Read the model definition and answer for the solid it produces. Units are mm, in the model's axes. A direction names the side the tool comes from. Give positions to 0.01 mm unless a question says otherwise; leave off trailing zeros. Loops run counter-clockwise (first coordinate to the right, second up) from the corner with the lowest first, then second, coordinate; pieces in that order, holes last. Notation, with made-up numbers: (-36.75, -38.75) - (-8.75, -38.75) arc R30 cw to (-8.75, -14.75) - close; hole circle Ø3 at (89, -35). An arc over 180 degrees is marked (long way). Put each result on its own line as item: value. Start each with the question number.
1. For faces 5 (the flat face through (-103, 60.3, 8)), 6 (the flat face through (-158, -4.7, -6)), 7 (the flat face through (-158, 65, -6)), 8 (the cylindrical face through (-139.866, -12.61, 17.484)), determine the directions among +Z, -Z, +X, -X, +Y, -Y from which every point of the face is accessible in a straight line to the end or side of a thin tool.
2. A cutting plane is placed at A-A, the plane y = 44.5. Determine the outline of the cut face in (x, z), plus the area to 3 significant figures.
3. A cutting plane is placed at D-D, the plane z = -4.3. Determine the outline of the cut face in (x, y).
4. A cutting plane is placed at B-B, the plane x = -111. Count the separate pieces of the cut face and the enclosed holes in it, plus the area to 3 significant figures.
5. For a pull along X with two mould halves and no side action, classify faces 1 (the flat face through (-111, 60, 0.8)), 2 (the flat face through (-100.01, 65.4, 10.88)), 3 (the flat face through (-150.9, 31, -4)), 4 (the flat face through (-159, 59, -3)) as released by +X, released by -X, zero draft, split by the parting line, or undercut.
6. A cutting plane is placed at C-C, the plane y = 5.2. Determine the outline of the cut face in (x, z), plus the area to 3 significant figures.
7. Consider L1, parallel to Y at x = -144.7, z = 0.95; L2, parallel to Y at x = -134, z = 20.5; L3, parallel to Y at x = -144, z = 1. Determine where each line is inside the solid, lowest interval first. Write a range as from..to.
8. Given pin 1 Ø1 at (y, z) = (60.5, 18) entering from -X; pin 2 Ø1.2 at (x, y) = (-102, 63) entering from +Z; pin 3 Ø7 at (x, z) = (-127.5, 9) entering from -Y; pin 4 Ø1.5 at (y, z) = (67, 11) entering from +X, each flat-ended and moving along its own axis, determine where each tip first touches the part or whether it passes through.
```python
from build123d import *

# Parameters (mm, degrees)
SKETCH_1_W          = 33.55
SKETCH_1_H          = 60.3
SKETCH_1_R          = 1.2
EXTRUDE_1_DEPTH     = 2
SKETCH_2_W          = 2
SKETCH_2_H          = 60.3
EXTRUDE_2_DEPTH     = 9.9
SKETCH_3_W          = 9.9
SKETCH_3_H          = 2
EXTRUDE_3_DEPTH     = 1.9
SKETCH_4_W          = 10.719852834
SKETCH_4_H          = 56.3
SKETCH_4_W_2        = 2
SKETCH_4_H_2        = 60.3
EXTRUDE_5_DEPTH     = 3
SKETCH_6_W          = 14.719852834
SKETCH_6_H          = 4.7
EXTRUDE_6_DEPTH     = 3
SKETCH_7_W          = 9.4
SKETCH_7_H          = 6
SKETCH_7_R          = 1.5
EXTRUDE_7_DEPTH     = 14.4
EXTRUDE_8_DEPTH     = 17.1
EXTRUDE_9_DEPTH     = 8.35
SKETCH_10_W         = 43.45
SKETCH_10_H         = 4
EXTRUDE_10_DEPTH    = 8.35
CUT_EXTRUDE_START   = -0.6
CUT_EXTRUDE_1_DEPTH = 0.6
CUT_EXTRUDE_2_DEPTH = 0.6
SKETCH_13_W         = 43.45
SKETCH_13_H         = 4
EXTRUDE_11_DEPTH    = 2
SKETCH_14_W         = 43.45
SKETCH_14_H         = 4
EXTRUDE_12_DEPTH    = 2
EXTRUDE_13_DEPTH    = 4
SKETCH_16_W         = 2.5
SKETCH_16_H         = 40
EXTRUDE_14_DEPTH    = 10
SKETCH_17_W         = 4
SKETCH_17_H         = 5.65
EXTRUDE_15_DEPTH    = 17.4
EXTRUDE_16_DEPTH    = 4
SKETCH_19_W         = 1.8
SKETCH_19_H         = 1.8
EXTRUDE_17_DEPTH    = 21.4
SKETCH_20_W         = 12.1
SKETCH_20_H         = 1.8
EXTRUDE_18_DEPTH    = 16
EXTRUDE_START       = -4
EXTRUDE_22_DEPTH    = 25.4
EXTRUDE_23_DEPTH    = 25.4
CUT_EXTRUDE_3_DEPTH = 21.4
EXTRUDE_24_DEPTH    = 4
EXTRUDE_25_DEPTH    = 21.4
SKETCH_26_W         = 1.445945033
SKETCH_26_H         = 2.5
EXTRUDE_26_DEPTH    = 10
EXTRUDE_27_DEPTH    = 21.4
EXTRUDE_28_DEPTH    = 21.4
SKETCH_29_W         = 21.4
SKETCH_29_H         = 5
EXTRUDE_29_DEPTH    = 3
SKETCH_30_R         = 1.2
CUT_EXTRUDE_4_DEPTH = 12
SKETCH_31_W         = 13.445945033
SKETCH_31_H         = 37.5
SKETCH_31_W_2       = 7.004054967
SKETCH_31_H_2       = 40
CUT_EXTRUDE_5_DEPTH = 2
CUT_EXTRUDE_START_2 = -9.4
CUT_EXTRUDE_6_DEPTH = 9.4
CHAMFER_2_SIZE      = 2
CHAMFER_3_SIZE      = 3
CHAMFER_4_SIZE      = 3


with BuildPart() as part:
    # 草图1 → 凸台-拉伸1 (new body)
    with BuildSketch(Plane.XY):
        with Locations((-131.125, 30.15)):
            Rectangle(SKETCH_1_W, SKETCH_1_H)
        with Locations((-144.7, 5.2)):
            Circle(SKETCH_1_R, mode=Mode.SUBTRACT)
        with Locations((-117.55, 5.2)):
            Circle(SKETCH_1_R, mode=Mode.SUBTRACT)
        with Locations((-117.55, 55.1)):
            Circle(SKETCH_1_R, mode=Mode.SUBTRACT)
        with Locations((-144.7, 55.1)):
            Circle(SKETCH_1_R, mode=Mode.SUBTRACT)
    extrude(amount=EXTRUDE_1_DEPTH)

    # 草图2 → 凸台-拉伸2 (add)
    with BuildSketch(Plane(origin=(-114.35, 0, 0), x_dir=(0, 0, -1), z_dir=(1, 0, 0))):
        with Locations((-1, 30.15)):
            Rectangle(SKETCH_2_W, SKETCH_2_H)
    extrude(amount=EXTRUDE_2_DEPTH)

    # 草图3 → 凸台-拉伸3 (add)
    with BuildSketch(Plane(origin=(0, 0, 0), x_dir=(-1, 0, 0), z_dir=(0, 0, -1))):
        with Locations((109.4, 59.3)):
            Rectangle(SKETCH_3_W, SKETCH_3_H)
        with Locations((109.4, 1)):
            Rectangle(SKETCH_3_W, SKETCH_3_H)
    extrude(amount=EXTRUDE_3_DEPTH)

    # 草图4 → 凸台-拉伸5 (add)
    with BuildSketch(Plane.ZY.offset(147.9)):
        Polygon((0, 60.3), (-12.719852834, 60.3), (-12.719852834, 58.3), (-2, 58.3), (-2, 2), (-12.719852834, 2), (-12.719852834, 0), (0, 0), align=None)
        with Locations((-7.359926417, 30.15)):
            Rectangle(SKETCH_4_W, SKETCH_4_H)
        with Locations((1, 30.15)):
            Rectangle(SKETCH_4_W_2, SKETCH_4_H_2)
    extrude(amount=EXTRUDE_5_DEPTH)

    # 草图6 → 凸台-拉伸6 (add)
    with BuildSketch(Plane.ZY.offset(150.9)):
        with Locations((-5.359926417, 62.65)):
            Rectangle(SKETCH_6_W, SKETCH_6_H)
        with Locations((-5.359926417, -2.35)):
            Rectangle(SKETCH_6_W, SKETCH_6_H)
    extrude(amount=-EXTRUDE_6_DEPTH)

    # 草图7 → 凸台-拉伸7 (add)
    # profile 1 of 2: a face of its own
    with BuildSketch(Plane.ZY.offset(150.9)):
        with Locations((-2.7, 62)):
            Rectangle(SKETCH_7_W, SKETCH_7_H)
        with Locations(Location((-4.3, 61.9, 0), (0, 0, 180))):
            Circle(SKETCH_7_R, mode=Mode.SUBTRACT)
    # profile 2 of 2: a face of its own
    with BuildSketch(Plane.ZY.offset(150.9)):
        with Locations((-2.7, -1.7)):
            Rectangle(SKETCH_7_W, SKETCH_7_H)
        with Locations(Location((-4.3, -1.6, 0), (0, 0, 180))):
            Circle(SKETCH_7_R, mode=Mode.SUBTRACT)
    extrude(amount=EXTRUDE_7_DEPTH)

    # 草图8 → 凸台-拉伸8 (add)
    with BuildSketch(Plane.ZY.offset(150.9)):
        Polygon((-7.8, 59), (-7.8, 1.3), (-7.4, 1.3), (-7.4, -4.7), (-12.719852834, -4.7), (-12.719852834, 65), (-7.4, 65), (-7.4, 59), align=None)
    extrude(amount=EXTRUDE_8_DEPTH)

    # 草图9 → 凸台-拉伸9 (add)
    with BuildSketch(Plane(origin=(0, 60.3, 0), x_dir=(1, 0, 0), z_dir=(0, 1, 0))):
        Polygon((-114.35, 1.9), (-114.35, 0), (-147.9, 0), (-147.9, -2), (-104.45, -2), (-104.45, 1.9), align=None)
        Polygon((-114.35, 1.9), (-104.45, 1.9), (-104.45, 2), (-147.9, 2), (-147.9, 0), (-114.35, 0), align=None)
    extrude(amount=EXTRUDE_9_DEPTH)

    # 草图10 → 凸台-拉伸10 (add)
    with BuildSketch(Plane.XZ):
        with Locations((-126.175, 0)):
            Rectangle(SKETCH_10_W, SKETCH_10_H)
    extrude(amount=EXTRUDE_10_DEPTH)

    # 草图11 → 切除-拉伸1 (cut)
    with BuildSketch(Plane.XY.offset(2).offset(CUT_EXTRUDE_START)):
        with BuildLine():
            Line((-104.45, 51.65), (-104.45, 67.75))
            Line((-104.45, 67.75), (-116.55, 67.75))
            Line((-116.55, 67.75), (-116.55, 55.763324958))
            ThreePointArc((-116.55, 55.763324958), (-116.354567134, 55.204595711), (-116.45, 54.620416848))
            Line((-116.45, 54.620416848), (-116.45, 51.65))
            Line((-116.45, 51.65), (-104.45, 51.65))
        make_face()
    extrude(amount=CUT_EXTRUDE_1_DEPTH, mode=Mode.SUBTRACT)

    # 草图12 → 切除-拉伸2 (cut)
    with BuildSketch(Plane.XY.offset(1.4)):
        with BuildLine():
            Line((-113.374176728, 54.65), (-107.45, 54.65))
            Line((-107.45, 54.65), (-107.45, 64.75))
            Line((-107.45, 64.75), (-113.55, 64.75))
            Line((-113.55, 64.75), (-113.55, 56.380624847))
            ThreePointArc((-113.55, 56.380624847), (-113.371508988, 55.524514858), (-113.374176728, 54.65))
        make_face()
    extrude(amount=-CUT_EXTRUDE_2_DEPTH, mode=Mode.SUBTRACT)

    # 草图13 → 凸台-拉伸11 (add)
    with BuildSketch(Plane(origin=(0, 68.65, 0), x_dir=(1, 0, 0), z_dir=(0, 1, 0))):
        with Locations((-126.175, 0)):
            Rectangle(SKETCH_13_W, SKETCH_13_H)
    extrude(amount=EXTRUDE_11_DEPTH)

    # 草图14 → 凸台-拉伸12 (add)
    with BuildSketch(Plane.XZ.offset(8.35)):
        with Locations((-126.175, 0)):
            Rectangle(SKETCH_14_W, SKETCH_14_H)
    extrude(amount=EXTRUDE_12_DEPTH)

    # 草图15 → 凸台-拉伸13 (add)
    with BuildSketch(Plane.XY.offset(2)):
        Polygon((-147.9, 70.65), (-165.3, 65), (-147.9, 65), align=None)
    extrude(amount=-EXTRUDE_13_DEPTH)

    # 草图16 → 凸台-拉伸14 (add)
    with BuildSketch(Plane.XY.offset(2)):
        with Locations((-142.645945033, 30.15)):
            Rectangle(SKETCH_16_W, SKETCH_16_H)
        with Locations((-119.145945033, 30.15)):
            Rectangle(SKETCH_16_W, SKETCH_16_H)
    extrude(amount=EXTRUDE_14_DEPTH)

    # 草图17 → 凸台-拉伸15 (add)
    with BuildSketch(Plane.ZY.offset(147.9)):
        with Locations((0, -7.525)):
            Rectangle(SKETCH_17_W, SKETCH_17_H)
    extrude(amount=EXTRUDE_15_DEPTH)

    # 草图18 → 凸台-拉伸16 (add)
    with BuildSketch(Plane.XY.offset(2)):
        Polygon((-104.45, 67.75), (-104.45, 60.3), (-95.7, 60.3), (-104.45, 70.65), align=None)
        Polygon((-104.45, 0), (-104.45, -10.35), (-95.7, 0), align=None)
    extrude(amount=-EXTRUDE_16_DEPTH)

    # 草图19 → 凸台-拉伸17 (add)
    with BuildSketch(Plane.XY.offset(2)):
        Polygon((-165.3, 65), (-159.471717964, 65), (-147.615080796, 68.85), (-118.35, 68.85), (-118.35, 70.65), (-147.9, 70.65), align=None)
        with Locations((-117.45, 69.75)):
            Rectangle(SKETCH_19_W, SKETCH_19_H)
        Polygon((-95.7, 60.3), (-104.45, 70.65), (-104.45, 67.861945247), (-102.65, 65.73280239), (-99.57879025, 62.1), (-99.57879025, 60.3), align=None)
        Polygon((-105.285311989, -8.55), (-163.5, -8.55), (-165.3, -8.55), (-165.3, -10.35), (-104.45, -10.35), (-95.7, 0), (-99.57879025, 0), (-99.57879025, -1.8), align=None)
    extrude(amount=EXTRUDE_17_DEPTH)

    # 草图20 → 凸台-拉伸18 (add)
    with BuildSketch(Plane.XY.offset(23.4)):
        with Locations((-110.5, 69.75)):
            Rectangle(SKETCH_20_W, SKETCH_20_H)
    extrude(amount=-EXTRUDE_18_DEPTH)

    # 草图21 → 凸台-拉伸22 (add)
    with BuildSketch(Plane.XY.offset(2).offset(EXTRUDE_START)):
        Polygon((-165.3, -8.55), (-165.3, -4.7), (-168, -4.7), (-165.3, -10.35), align=None)
    extrude(amount=EXTRUDE_22_DEPTH)

    # 草图22 → 凸台-拉伸23 (add)
    with BuildSketch(Plane.XY.offset(23.4)):
        Polygon((-163.305030212, -10.35), (-165.3, -10.35), (-162.432743363, -16.35), (-141.174369577, -16.35), (-137.174369577, -10.35), (-138.374369577, -10.35), (-141.174369577, -14.55), (-161.297950566, -14.55), align=None)
    extrude(amount=-EXTRUDE_23_DEPTH)

    # 草图23 → 切除-拉伸3 (cut)
    with BuildSketch(Plane.XY.offset(23.4)):
        Polygon((-164.165207203, -8.55), (-163.305030212, -10.35), (-138.374369577, -10.35), (-137.174369577, -8.55), align=None)
    extrude(amount=-CUT_EXTRUDE_3_DEPTH, mode=Mode.SUBTRACT)

    # 草图24 → 凸台-拉伸24 (add)
    with BuildSketch(Plane(origin=(0, 0, -2), x_dir=(-1, 0, 0), z_dir=(0, 0, -1))):
        Polygon((141.174369577, -14.55), (161.297950566, -14.55), (163.305030212, -10.35), (138.374369577, -10.35), align=None)
    extrude(amount=-EXTRUDE_24_DEPTH)

    # 草图25 → 凸台-拉伸25 (add)
    with BuildSketch(Plane.XY.offset(2)):
        Polygon((-147.615080796, 68.85), (-149.4421323, 68.256733276), (-149.4421323, 63.85), (-144.4421323, 63.85), (-144.4421323, 68.85), align=None)
        Polygon((-141.174369577, -8.55), (-141.174369577, -14.55), (-137.174369577, -8.55), align=None)
        Polygon((-105.285311989, 0), (-104.45, 0), (-99.57879025, 0), (-99.57879025, -1.8), (-105.285311989, -8.55), align=None)
    extrude(amount=EXTRUDE_25_DEPTH)

    # 草图26 → 凸台-拉伸26 (add)
    with BuildSketch(Plane.XY.offset(2)):
        Polygon((-116.45, 50.15), (-116.45, 47.65), (-104.45, 47.65), (-104.45, 51.65), (-116.45, 51.65), align=None)
        with Locations((-117.172972517, 48.9)):
            Rectangle(SKETCH_26_W, SKETCH_26_H)
    extrude(amount=EXTRUDE_26_DEPTH)

    # 草图27 → 凸台-拉伸27 (add)
    with BuildSketch(Plane.XY.offset(2)):
        Polygon((-104.45, 67.861945247), (-104.45, 67.75), (-104.45, 60.3), (-99.57879025, 60.3), (-99.57879025, 62.1), align=None)
    extrude(amount=EXTRUDE_27_DEPTH)

    # 草图28 → 凸台-拉伸28 (add)
    with BuildSketch(Plane.XY.offset(23.4)):
        Polygon((-141.174369577, -14.55), (-141.174369577, -8.55), (-145.174369577, -14.55), align=None)
    extrude(amount=-EXTRUDE_28_DEPTH)

    # 草图29 → 凸台-拉伸29 (add)
    with BuildSketch(Plane(origin=(-144.4421323, 0, 0), x_dir=(0, 0, -1), z_dir=(1, 0, 0))):
        with Locations((-12.7, 66.35)):
            Rectangle(SKETCH_29_W, SKETCH_29_H)
    extrude(amount=EXTRUDE_29_DEPTH)

    # 草图30 → 切除-拉伸4 (cut)
    with BuildSketch(Plane.XY.offset(23.4)):
        with Locations((-102.285311989, -3.2)):
            Circle(SKETCH_30_R)
        with Locations((-101.45, 63.5)):
            Circle(SKETCH_30_R)
        with Locations((-140.974369577, -12.15)):
            Circle(SKETCH_30_R)
        with Locations((-145.6421323, 67.45)):
            Circle(SKETCH_30_R)
    extrude(amount=-CUT_EXTRUDE_4_DEPTH, mode=Mode.SUBTRACT)

    # 草图31 → 切除-拉伸5 (cut)
    with BuildSketch(Plane.XY.offset(2)):
        with Locations((-111.172972517, 28.9)):
            Rectangle(SKETCH_31_W, SKETCH_31_H)
        with Locations((-147.397972517, 30.15)):
            Rectangle(SKETCH_31_W_2, SKETCH_31_H_2)
    extrude(amount=-CUT_EXTRUDE_5_DEPTH, mode=Mode.SUBTRACT)

    # 草图32 → 切除-拉伸6 (cut)
    with BuildSketch(Plane.XY.offset(12).offset(CUT_EXTRUDE_START_2)):
        Polygon((-117.895945033, 50.15), (-117.895945033, 47.65), (-104.45, 47.65), (-104.45, 51.65), (-116.45, 51.65), (-116.45, 50.15), align=None)
    extrude(amount=CUT_EXTRUDE_6_DEPTH, mode=Mode.SUBTRACT)

    # 倒角2
    chamfer_2_edges = [part.edges().sort_by_distance(p)[0] for p in [
        (-126.175, 70.65, -2),
        (-120.812184789, -10.35, -2),
        (-151.80355647, -16.35, -2),
    ]]
    chamfer(chamfer_2_edges, length=CHAMFER_2_SIZE)

    # 倒角3
    chamfer_3_edges = [part.edges().sort_by_distance(p)[0] for p in [
        (-157.95, -4.7, -12.719852834),
        (-157.95, 65, -12.719852834),
    ]]
    chamfer(chamfer_3_edges, length=CHAMFER_3_SIZE)

    # 倒角4
    chamfer_4_edges = [part.edges().sort_by_distance(p)[0] for p in [
        (-168, 30.15, -12.719852834),
    ]]
    chamfer(chamfer_4_edges, length=CHAMFER_4_SIZE)


solid = part.part
```
Return value:
1. face 5: -Z
1. face 6: -Z, +X, -X, -Y
1. face 7: -Z, +X, -X, +Y
1. face 8: +Z
2. outline: (-168, -9.72) - (-165, -12.72) - (-147.9, -12.72) - (-147.9, 0) - (-150.9, 0) - (-150.9, -7.8) - (-168, -7.8) - close; (-143.9, 0) - (-117.9, 0) - (-117.9, 12) - (-120.4, 12) - (-120.4, 2) - (-141.4, 2) - (-141.4, 12) - (-143.9, 12) - close
2. area: 220 mm2
3. outline: (-165.3, -4.7) - (-147.9, -4.7) - (-147.9, 65) - (-165.3, 65) - (-165.3, 63.4) - (-150.9, 63.4) - (-150.9, 60.4) - (-165.3, 60.4) - (-165.3, 59) - (-150.9, 59) - (-150.9, 1.3) - (-165.3, 1.3) - (-165.3, -0.1) - (-150.9, -0.1) - (-150.9, -3.1) - (-165.3, -3.1) - close
4. separate pieces: 3
4. enclosed holes: 0
4. area: 186 mm2
5. face 1: undercut
5. face 2: released by +X
5. face 3: released by -X
5. face 4: zero draft
6. outline: (-168, -9.72) - (-165, -12.72) - (-147.9, -12.72) - (-147.9, 0) - (-145.9, 0) - (-145.9, 2) - (-150.9, 2) - (-150.9, -7.8) - (-168, -7.8) - close; (-143.5, 0) - (-118.75, 0) - (-118.75, 2) - (-143.5, 2) - close; (-116.35, 0) - (-104.45, 0) - (-104.45, 2) - (-116.35, 2) - close
6. area: 201 mm2
7. L1: y = -16.35..4, 6.4..10.15, 50.15..53.9, 56.3..70.65
7. L2: y = -10.35..-8.55, 68.85..70.65
7. L3: y = -16.35..4.23, 6.17..10.15, 50.15..54.13, 56.07..70.65
8. pin 1: stops at x = -104.45
8. pin 2: stops at z = 23.4
8. pin 3: stops at y = -10.35
8. pin 4: stops at x = -100.73
